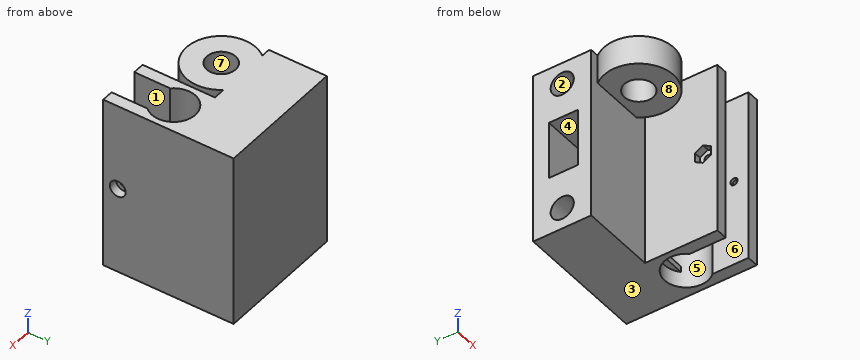
from build123d import *

# Parameters (mm, degrees)
SKETCH_W        = 45
SKETCH_H        = 60
PAD_DEPTH       = 20
SKETCH001_R     = 4
POCKET_DEPTH    = 40
SKETCH002_W     = 20
SKETCH002_H     = 10
POCKET001_DEPTH = 40
SKETCH003_W     = 19
SKETCH003_H     = 60
PAD001_DEPTH    = 25
POCKET002_DEPTH = 60
SKETCH005_W     = 19
SKETCH005_H     = 2
PAD002_DEPTH    = 2
SKETCH006_R     = 12
SKETCH006_R_2   = 5
PAD003_DEPTH    = 10
SKETCH007_R     = 1.25
POCKET003_DEPTH = 45.001
SKETCH008_R     = 2.75
POCKET004_DEPTH = 3
POCKET005_DEPTH = 2.4


with BuildPart() as part:
    # Sketch → Pad (new body)
    with BuildSketch(Plane.XZ):
        Rectangle(SKETCH_W, SKETCH_H)
    extrude(amount=PAD_DEPTH)

    # Sketch001 (on Face4 of Pad) → Pocket (cut)
    with BuildSketch(Plane(origin=(-22.5, 0, 0), x_dir=(0, 0, -1), z_dir=(-1, 0, 0))):
        with Locations((-22.5, 10)):
            Circle(SKETCH001_R)
        with Locations((22.5, 10)):
            Circle(SKETCH001_R)
    extrude(amount=-POCKET_DEPTH, mode=Mode.SUBTRACT)

    # Sketch002 (on Face2 of Pocket) → Pocket001 (cut)
    with BuildSketch(Plane(origin=(-22.5, 0, 0), x_dir=(0, 0, -1), z_dir=(-1, 0, 0))):
        with Locations((-0.462425, 10.424613)):
            Rectangle(SKETCH002_W, SKETCH002_H)
    extrude(amount=-POCKET001_DEPTH, mode=Mode.SUBTRACT)

    # Sketch003 (on Face5 of Pocket001) → Pad001 (join)
    with BuildSketch(Plane.XZ.offset(20)):
        with Locations((13, 0)):
            Rectangle(SKETCH003_W, SKETCH003_H)
    extrude(amount=PAD001_DEPTH)

    # Sketch004 (on Face6 of Pad001) → Pocket002 (cut)
    with BuildSketch(Plane(origin=(0, 0, 30), x_dir=(-1, 0, 0), z_dir=(0, 0, 1))):
        with BuildLine():
            Line((-18.5, 45), (-7.5, 45))
            Line((-7.5, 45), (-7.5, 32.59902))
            ThreePointArc((-18.5, 32.59902), (-13, 20), (-7.5, 32.59902))
            Line((-18.5, 32.59902), (-18.5, 45))
        make_face()
    extrude(amount=-POCKET002_DEPTH, mode=Mode.SUBTRACT)

    # Sketch005 (on Face4 of Pocket002) → Pad002 (join)
    with BuildSketch(Plane.XZ.offset(20)):
        with Locations((13, 23.5)):
            Rectangle(SKETCH005_W, SKETCH005_H)
        with Locations((13, -23.5)):
            Rectangle(SKETCH005_W, SKETCH005_H)
    extrude(amount=PAD002_DEPTH)

    # Sketch006 (on Face1 of Pad002) → Pad003 (join)
    with BuildSketch(Plane(origin=(0, 0, 30), x_dir=(-1, 0, 0), z_dir=(0, 0, 1))):
        with Locations((10, 27.5)):
            Circle(SKETCH006_R)
        with Locations((10, 27.5)):
            Circle(SKETCH006_R_2, mode=Mode.SUBTRACT)
    extrude(amount=-PAD003_DEPTH)

    # Sketch007 (on Face10 of Pad003) → Pocket003 (cut, through all)
    with BuildSketch(Plane(origin=(22.5, 0, 0), x_dir=(0, 0, 1), z_dir=(1, 0, 0))):
        with Locations((0, 40)):
            Circle(SKETCH007_R)
    extrude(amount=-POCKET003_DEPTH, mode=Mode.SUBTRACT)

    # Sketch008 (on Face10 of Pocket003) → Pocket004 (cut)
    with BuildSketch(Plane(origin=(22.5, 0, 0), x_dir=(0, 0, 1), z_dir=(1, 0, 0))):
        with Locations((0, 40)):
            Circle(SKETCH008_R)
    extrude(amount=-POCKET004_DEPTH, mode=Mode.SUBTRACT)

    # Sketch009 (on Face18 of Pocket004) → Pocket005 (cut)
    with BuildSketch(Plane(origin=(3.5, 0, 0), x_dir=(0, 0, -1), z_dir=(-1, 0, 0))):
        Polygon((1.587713, 37.25), (3.175426, 40), (1.587713, 42.75), (-1.587713, 42.75), (-3.175426, 40), (-1.587713, 37.25), align=None)
    extrude(amount=-POCKET005_DEPTH, mode=Mode.SUBTRACT)


solid = part.part
For this review, take the finished solid that the model builds, in its own axes (mm). Face numbers are marked on the shaded views. A direction names the side the tool comes from. Coordinates: 2 decimals unless noted, no trailing zeros. Loops run counter-clockwise (first coordinate to the right, second up) from the corner with the lowest first, then second, coordinate; pieces in that order, holes last. Notation, with made-up numbers: (28, 7.5) - (77, 7.5) arc R18 cw to (77, 21.5) - close; hole circle Ø8 at (6.5, 26.25). An arc over 180 degrees is marked (long way). Return JSON: item names as keys, results as strings.
Item 1: Take a section at B-B (y = -27.5). Give the boundary of the cut face in (x, z), then the cut area to 3 significant figures.
Determined:
{"outline": "(-22, 20) - (-15, 20) - (-15, 30) - (-22, 30) - close; (-5, 20) - (2, 20) - (2, 30) - (-5, 30) - close; (3.5, -30) - (5.5, -30) - (5.5, 30) - (3.5, 30) - close; (20.5, -30) - (22.5, -30) - (22.5, 30) - (20.5, 30) - close", "area": "380 mm2"}
Item 2: Mouldability with a two-part tool opening along Z and no side actions: class the marked faces 1, 2 and 3 as pulls with the +Z half, pulls with the -Z half, needs draft (parallel to the pull), parting line crosses it, or undercut.
Determined:
{"face 1": "needs draft", "face 2": "undercut", "face 3": "pulls with the -Z half"}
Item 3: Take a section at A-A (x = -10). Give the boundary of the cut face in (y, z), then the cut area to 3 significant figures.
Determined:
{"outline": "(-39.5, 20) - (-32.5, 20) - (-32.5, 30) - (-39.5, 30) - close; (-22.5, 20) - (-20, 20) - (-20, -30) - (0, -30) - (0, 30) - (-22.5, 30) - close; hole (-15.42, -9.54) - (-5.42, -9.54) - (-5.42, 10.46) - (-15.42, 10.46) - close; hole circle Ø8 at (-10, -22.5); hole circle Ø8 at (-10, 22.5)", "area": "994 mm2"}
Item 4: Insertion check: pin 1 (5 mm diameter, centred on y = -39, z = -8.5, fed in from -X); pin 2 (2 mm diameter, centred on y = -40, z = 0, fed in from +X); pin 3 (4 mm diameter, centred on y = -9.5, z = -21, fed in from -X); pin 4 (0.6 mm diameter, centred on x = 12, y = -20.5, fed in from -Z). Each pin has a flat end and moves straight along its axis. Give the tip position at first contact, or say it passes through.
Determined:
{"pin 1": "stops at x = 3.5", "pin 2": "passes through", "pin 3": "stops at x = 17.5", "pin 4": "stops at z = -24.5"}
Item 5: For the marked faces 4, 5, 6, 7 and 8, list the 3-axis set-ups (+Z, -Z, +X, -X, +Y, -Y) from which the entire face can be reached by the end or side of a thin tool; tool diameter is ignored.
Determined:
{"face 4": "-X", "face 5": "none", "face 6": "+Z, -Z, -Y", "face 7": "+Z, -Z", "face 8": "-Z, -X, -Y"}
Item 6: Take a section at C-C (z = 0). State how many separate pieces and enclosed holes the cut face has, then the cut area to 3 significant figures.
Determined:
{"separate pieces": "3", "enclosed holes": "0", "area": "644 mm2"}
Item 7: For line 1 (Z direction, x = -14, y = -10); line 2 (Y direction, x = 21.1, z = 0); line 3 (Z direction, x = 19.2, y = -40), list the stretches that pass through material, from the lowest coordinate up.
Determined:
{"line 1": "z = -30 to -26.5, -18.5 to -9.54, 10.46 to 18.5, 26.5 to 30", "line 2": "y = -45 to -42.75, -37.25 to 0", "line 3": "z = -30 to -1.25, 1.25 to 30"}
Item 8: Take a section at D-D (x = 13). Give the boundary of the cut face in (y, z).
Determined:
{"outline": "(-22, -24.5) - (-20, -24.5) - (-20, -30) - (0, -30) - (0, 30) - (-20, 30) - (-20, 24.5) - (-22, 24.5) - (-22, 22.5) - (-20, 22.5) - (-20, -22.5) - (-22, -22.5) - close; hole (-15.42, -9.54) - (-5.42, -9.54) - (-5.42, 10.46) - (-15.42, 10.46) - close; hole circle Ø8 at (-10, -22.5); hole circle Ø8 at (-10, 22.5)"}
